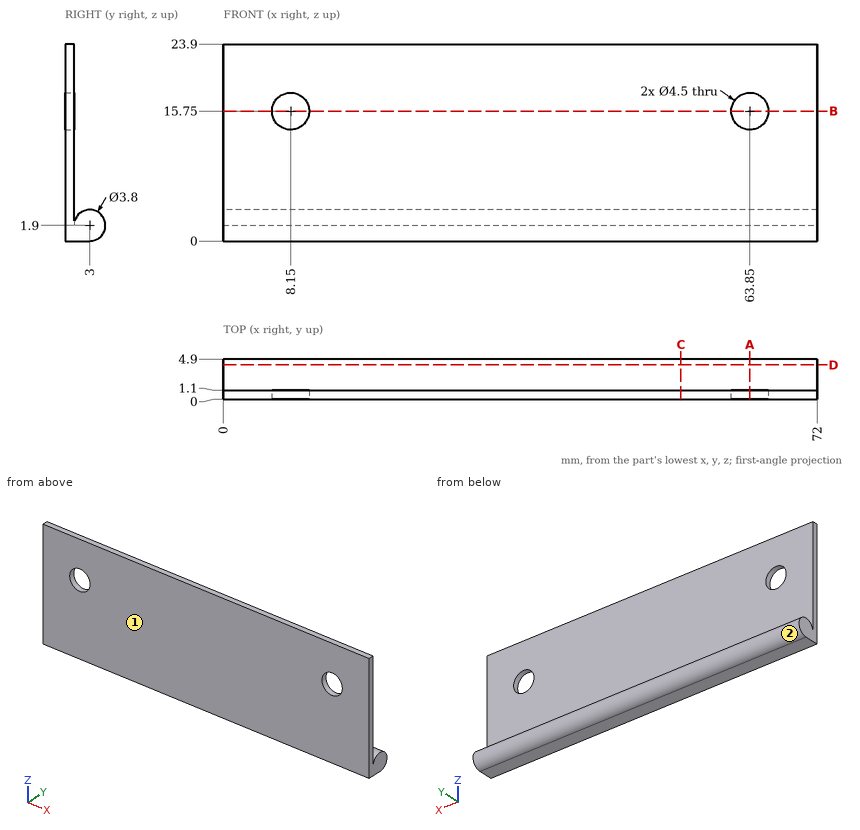
Can you work these out from the drawing? Everything is in mm from the part's minimum corner. Round coordinates to 2 decimals unless told otherwise and drop trailing zeros. Order: outer loops, then holes, each group sorted by start corner. A loop starts at its lowest first (then second) coordinate and runs counter-clockwise, first axis right, second up. Notation, with made-up numbers: (-20.75, -24) -> (2.25, -24) arc R25 cw to (2.25, -4) -> close; hole circle Ø11 at (69.25, 87.5). An arc over 180 degrees is marked (long way). Use CSV: the item, a comma, the result in double quotes.
1. I need wall thicknesses on line 1 along X through (y, z) = (0.6, 15.75); line 2 along Z through (x, y) = (63.85, 0.4); line 3 along Y through (x, z) = (68.5, 16.75). Which ranges of each line are inside material? Lowest first, please.
Recorded:
line 1,"x = 0 to 5.9, 10.4 to 61.6, 66.1 to 72"
line 2,"z = 0 to 13.5, 18 to 23.9"
line 3,"y = 0 to 1.1"
2. Thinking about a two-plate mould opening in Y: for the marked faces 1 and 2, which applies, pulls with the +Y half, pulls with the -Y half, needs draft (parallel to the pull), parting line crosses it, or undercut?
Recorded:
face 1,"pulls with the -Y half"
face 2,"undercut"
3. I want a section at C-C on x = 55.5. List the corners of the cut face in (y, z) for me.
Recorded:
outline,"(0, 0) -> (3, 0) arc R1.9 ccw (long way) to (1.1, 1.9) -> (1.1, 23.9) -> (0, 23.9) -> close"
4. I'm going to push flat-ended pins straight in: P1, Ø2, axis at x = 33, z = 6.5, coming from the -Y side; P2, Ø8, axis at x = 16, z = 20, coming from the +Y side. Where does each tip first touch, or does it pass through?
Recorded:
P1,"stops at y = 0"
P2,"stops at y = 1.1"
5. I want a section at D-D on y = 4.2. List the corners of the cut face in (x, z) for me.
Recorded:
outline,"(0, 0.43) -> (72, 0.43) -> (72, 3.37) -> (0, 3.37) -> close"
6. I want a section at B-B on z = 15.75. List the corners of the cut face in (x, y) for me, and give its area (3 significant figures).
Recorded:
outline,"(0, 0) -> (5.9, 0) -> (5.9, 1.1) -> (0, 1.1) -> close; (10.4, 0) -> (61.6, 0) -> (61.6, 1.1) -> (10.4, 1.1) -> close; (66.1, 0) -> (72, 0) -> (72, 1.1) -> (66.1, 1.1) -> close"
area,"69.3 mm2"
7. I want a section at A-A on x = 63.85. List the corners of the cut face in (y, z) for me.
Recorded:
outline,"(0, 0) -> (3, 0) arc R1.9 ccw (long way) to (1.1, 1.9) -> (1.1, 13.5) -> (0, 13.5) -> close; (0, 18) -> (1.1, 18) -> (1.1, 23.9) -> (0, 23.9) -> close"
